```python
from build123d import *

# Parameters (mm, degrees)
F1_DEPTH = 1
F2_R     = 0.9
F3_DEPTH = 5
F4_DEPTH = 1.001


with BuildPart() as f1:
    # F0 (on Top) → F1 (new body)
    with BuildSketch(Plane.XY):
        with BuildLine():
            ThreePointArc((-96.1861413951, -113.2155081954), (-68.1861413951, -141.2155081954), (-40.1861413951, -113.2155081954))
            Line((-40.1861413951, -113.2155081954), (-96.1861413951, -113.2155081954))
        make_face()
    extrude(amount=F1_DEPTH)

    # F2 (on face) → F3 (join)
    with BuildSketch(Plane.XY.offset(1)):
        with BuildLine():
            Line((-89.0189571251, -121.2155081954), (-95.0189571251, -121.2155081954))
            ThreePointArc((-95.0189571251, -121.2155081954), (-92.6129518517, -126.9023972105), (-89.0189571251, -131.9236291261))
            Line((-89.0189571251, -131.9236291261), (-89.0189571251, -121.2155081954))
        make_face()
        with Locations((-90.7189571251, -126.4236291261)):
            Circle(F2_R, mode=Mode.SUBTRACT)
        with Locations((-92.3189571251, -123.1155081954)):
            Circle(F2_R, mode=Mode.SUBTRACT)
        with BuildLine():
            Line((-47.3533256651, -121.2155081954), (-47.3533256651, -131.9236291261))
            ThreePointArc((-47.3533256651, -131.9236291261), (-43.7593309384, -126.9023972105), (-41.3533256651, -121.2155081954))
            Line((-41.3533256651, -121.2155081954), (-47.3533256651, -121.2155081954))
        make_face()
        with Locations((-45.6533256651, -126.4236291261)):
            Circle(F2_R, mode=Mode.SUBTRACT)
        with Locations((-44.0533256651, -123.1155081954)):
            Circle(F2_R, mode=Mode.SUBTRACT)
    extrude(amount=F3_DEPTH)

    # F2 (on face) → F4 (cut, through all)
    with BuildSketch(Plane.XY.offset(1)):
        with Locations((-92.3189571251, -123.1155081954)):
            Circle(F2_R)
        with Locations((-90.7189571251, -126.4236291261)):
            Circle(F2_R)
        with Locations((-44.0533256651, -123.1155081954)):
            Circle(F2_R)
        with Locations((-45.6533256651, -126.4236291261)):
            Circle(F2_R)
    extrude(amount=-F4_DEPTH, mode=Mode.SUBTRACT)


solid = f1.part
```
Input: part model. Units: mm. Frame: model coordinates. A direction names the side the tool comes from. Give positions to 0.01 mm unless a question says otherwise; leave off trailing zeros. Loops run counter-clockwise (first coordinate to the right, second up) from the corner with the lowest first, then second, coordinate; pieces in that order, holes last.
1) Contact query for flat-ended pins moving along their axis: pin 1 (2.5 mm diameter, centred on x = -45.5, z = 3.5, fed in from +Y); pin 2 (2.5 mm diameter, centred on x = -44.05, y = -123.12, fed in from -Z); pin 3 (1.6 mm diameter, centred on x = -90.72, y = -126.42, fed in from -Z); pin 4 (14 mm diameter, centred on x = -70.5, y = -121.5, fed in from +Z). Output: stop coordinate, or through.
A:
pin 1: stops at y = -121.22
pin 2: stops at z = 0
pin 3: passes through
pin 4: stops at z = 1
2) Reachability of faces 1 (the flat face through (-47.353, -126, 3)), 2 (the flat face through (-44, -121.216, 3)), 3 (the flat face through (-45, -125, 6)) from +Z, -Z, +X, -X, +Y, -Y: full face, straight path, thin tool, end or side. Return the list, or none.
A:
face 1: +Z, +Y, -Y
face 2: +Z, +X, -X, +Y
face 3: +Z, +X, -X, +Y, -Y
3) Section query B-B on y = -129.75. Return the cut outline in (x, z), and give its area (3 significant figures).
A:
outline: (-90.78, 0) - (-45.59, 0) - (-45.59, 6) - (-47.35, 6) - (-47.35, 1) - (-89.02, 1) - (-89.02, 6) - (-90.78, 6) - close
area: 62.8 mm2
4) Section query A-A on z = 4.2. Return the cut outline in (x, y), and give its area (3 significant figures).
A:
outline: (-95.02, -121.22) arc R28 ccw to (-89.02, -131.92) - (-89.02, -121.22) - close; (-47.35, -131.92) arc R28 ccw to (-41.35, -121.22) - (-47.35, -121.22) - close; hole circle Ø1.8 at (-92.32, -123.12); hole circle Ø1.8 at (-90.72, -126.42); hole circle Ø1.8 at (-45.65, -126.42); hole circle Ø1.8 at (-44.05, -123.12)
area: 65.2 mm2
5) Line query: L1, parallel to X at y = -122.5, z = 2.9; L2, parallel to Z at x = -66.5, y = -138.5; L3, parallel to Y at x = -91, z = 3.4. Output: solid intervals per line, ascending.
A:
L1: x = -94.6 to -92.98, -91.66 to -89.02, -47.35 to -44.71, -43.4 to -41.77
L2: z = 0 to 1
L3: y = -129.45 to -127.28, -125.57 to -121.22
6) Mould query, pull axis X, two halves, no side actions, for faces 4 (the flat face through (-69, -124, 0)), 5 (the flat face through (-89.019, -127, 3)). Classes: released by +X, released by -X, zero draft, split by the parting line, or undercut.
A:
face 4: zero draft
face 5: undercut
7) Section query C-C on x = -64. Return the cut outline in (y, z).
A:
outline: (-140.9, 0) - (-113.22, 0) - (-113.22, 1) - (-140.9, 1) - close
8) Section query D-D on y = -116.5. Return the cut outline in (x, z).
A:
outline: (-95.99, 0) - (-40.38, 0) - (-40.38, 1) - (-95.99, 1) - close
